Can you work these out from the model? Positions are in its coordinate system, mm. Face numbers are marked on the shaded views. Give positions to 0.01 mm unless a question says otherwise; leave off trailing zeros. Write each loop counter-clockwise with the first axis right and the second up, starting at its lowest first coordinate (ties: lowest second). Pieces come first, ordered by that corner, then holes. Notation, with made-up numbers: (34.25, 50.25) -> (57.25, 50.25) arc R25 ccw to (57.25, 83.25) -> close; hole circle Ø7 at (-22, 22). An arc over 180 degrees is marked (long way). One line per item, written item: value.
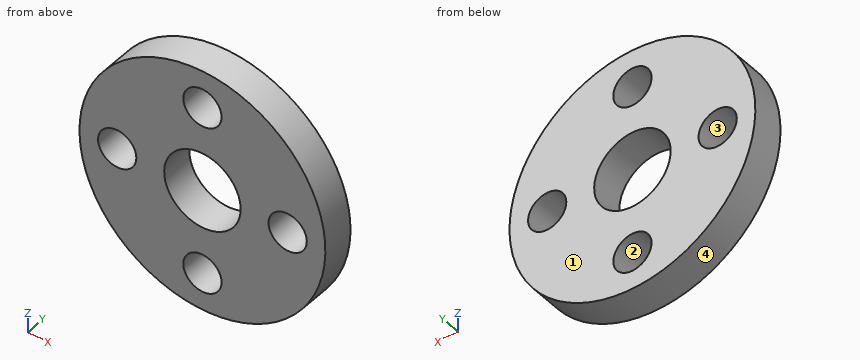
from build123d import *

# Parameters (mm, degrees)
SKETCH1_R           = 11.25
BOSS_EXTRUDE1_DEPTH = 3
CUT_EXTRUDE1_REACH  = 18.19
SKETCH2_R           = 1.75
SKETCH2_R_2         = 3.5


with BuildPart() as part:
    # Sketch1 → Boss-Extrude1 (new body)
    with BuildSketch(Plane(origin=(0, 0, 0), x_dir=(1, 0, 0), z_dir=(0, 1, 0))):
        with Locations(Location((0, 0, 0), (0, 0, 270))):
            Circle(SKETCH1_R)
    extrude(amount=BOSS_EXTRUDE1_DEPTH)

    # Sketch2 → Cut-Extrude1 (cut, up to next)
    with BuildSketch(Plane(origin=(0, 3, 0), x_dir=(1, 0, 0), z_dir=(0, 1, 0)), mode=Mode.PRIVATE) as cut_extrude1_sk1:
        with Locations(Location((0, 7.8, 0), (0, 0, 270))):
            Circle(SKETCH2_R)
    cut_extrude1_tool1 = extrude(cut_extrude1_sk1.sketch, amount=-CUT_EXTRUDE1_REACH, mode=Mode.PRIVATE) & part.part
    # Sketch2 → Cut-Extrude1 (cut, up to next)
    with BuildSketch(Plane(origin=(0, 3, 0), x_dir=(1, 0, 0), z_dir=(0, 1, 0)), mode=Mode.PRIVATE) as cut_extrude1_sk2:
        with Locations(Location((7.8, 0, 0), (0, 0, 270))):
            Circle(SKETCH2_R)
    cut_extrude1_tool2 = extrude(cut_extrude1_sk2.sketch, amount=-CUT_EXTRUDE1_REACH, mode=Mode.PRIVATE) & part.part
    # Sketch2 → Cut-Extrude1 (cut, up to next)
    with BuildSketch(Plane(origin=(0, 3, 0), x_dir=(1, 0, 0), z_dir=(0, 1, 0)), mode=Mode.PRIVATE) as cut_extrude1_sk3:
        with Locations(Location((0, -7.8, 0), (0, 0, 270))):
            Circle(SKETCH2_R)
    cut_extrude1_tool3 = extrude(cut_extrude1_sk3.sketch, amount=-CUT_EXTRUDE1_REACH, mode=Mode.PRIVATE) & part.part
    # Sketch2 → Cut-Extrude1 (cut, up to next)
    with BuildSketch(Plane(origin=(0, 3, 0), x_dir=(1, 0, 0), z_dir=(0, 1, 0)), mode=Mode.PRIVATE) as cut_extrude1_sk4:
        with Locations(Location((-7.8, 0, 0), (0, 0, 270))):
            Circle(SKETCH2_R)
    cut_extrude1_tool4 = extrude(cut_extrude1_sk4.sketch, amount=-CUT_EXTRUDE1_REACH, mode=Mode.PRIVATE) & part.part
    # Sketch2 → Cut-Extrude1 (cut, up to next)
    with BuildSketch(Plane(origin=(0, 3, 0), x_dir=(1, 0, 0), z_dir=(0, 1, 0)), mode=Mode.PRIVATE) as cut_extrude1_sk5:
        with Locations(Location((0, 0, 0), (0, 0, 270))):
            Circle(SKETCH2_R_2)
    cut_extrude1_tool5 = extrude(cut_extrude1_sk5.sketch, amount=-CUT_EXTRUDE1_REACH, mode=Mode.PRIVATE) & part.part
    add(cut_extrude1_tool1.solids().sort_by_distance((0, 3, -7.8))[0], mode=Mode.SUBTRACT)
    add(cut_extrude1_tool2.solids().sort_by_distance((7.8, 3, 0))[0], mode=Mode.SUBTRACT)
    add(cut_extrude1_tool3.solids().sort_by_distance((0, 3, 7.8))[0], mode=Mode.SUBTRACT)
    add(cut_extrude1_tool4.solids().sort_by_distance((-7.8, 3, 0))[0], mode=Mode.SUBTRACT)
    add(cut_extrude1_tool5.solids().sort_by_distance((0, 3, 0))[0], mode=Mode.SUBTRACT)


solid = part.part
1) I need wall thicknesses on L1, parallel to X at y = 0.75, z = 0; L2, parallel to Z at x = 9.25, y = 2.1; L3, parallel to Z at x = 0.5, y = 2.6. Which ranges of each line are inside material? Lowest first, please.
Answer list:
L1: x = -11.25 to -9.55, -6.05 to -3.5, 3.5 to 6.05, 9.55 to 11.25
L2: z = -6.4 to -0.98, 0.98 to 6.4
L3: z = -11.24 to -9.48, -6.12 to -3.46, 3.46 to 6.12, 9.48 to 11.24
2) We'd pull the mould along Z, two halves only. Please class the marked faces 1, 2, 3 and 4: released by +Z, released by -Z, zero draft, split by the parting line, or undercut.
Answer list:
face 1: zero draft
face 2: undercut
face 3: undercut
face 4: split by the parting line
3) If we section it at C-C (x = -2.25): Write out the boundary of the cut face in (y, z).
Answer list:
outline: (0, -11.02) -> (3, -11.02) -> (3, -2.68) -> (0, -2.68) -> close; (0, 2.68) -> (3, 2.68) -> (3, 11.02) -> (0, 11.02) -> close
4) If we section it at A-A (x = 0): Write out the boundary of the cut face in (y, z).
Answer list:
outline: (0, -11.25) -> (3, -11.25) -> (3, -9.55) -> (0, -9.55) -> close; (0, -6.05) -> (3, -6.05) -> (3, -3.5) -> (0, -3.5) -> close; (0, 3.5) -> (3, 3.5) -> (3, 6.05) -> (0, 6.05) -> close; (0, 9.55) -> (3, 9.55) -> (3, 11.25) -> (0, 11.25) -> close
5) Will this pin go through, and if not, where does the flat tip stop? pin 1 (1 mm diameter, centred on y = 1, z = -1, fed in from -X).
Answer list:
pin 1: stops at x = -11.24
6) If we section it at B-B (z = 0): Write out the boundary of the cut face in (x, y), and give its area (3 significant figures).
Answer list:
outline: (-11.25, 0) -> (-9.55, 0) -> (-9.55, 3) -> (-11.25, 3) -> close; (-6.05, 0) -> (-3.5, 0) -> (-3.5, 3) -> (-6.05, 3) -> close; (3.5, 0) -> (6.05, 0) -> (6.05, 3) -> (3.5, 3) -> close; (9.55, 0) -> (11.25, 0) -> (11.25, 3) -> (9.55, 3) -> close
area: 25.5 mm^2
7) If we section it at D-D (z = -7): Write out the boundary of the cut face in (x, y), and give its area (3 significant figures).
Answer list:
outline: (-8.81, 0) -> (-1.56, 0) -> (-1.56, 3) -> (-8.81, 3) -> close; (1.56, 0) -> (8.81, 0) -> (8.81, 3) -> (1.56, 3) -> close
area: 43.5 mm^2
